The listing builds one solid part. Answer for the finished solid, in the listing's coordinates (mm). Coordinates: 2 decimals unless noted, no trailing zeros. Order: outer loops, then holes, each group sorted by start corner. A loop starts at its lowest first (then second) coordinate and runs counter-clockwise, first axis right, second up.
from build123d import *

# Parameters (mm, degrees)
F0_W     = 279.4
F0_H     = 101.6
F1_DEPTH = 12.7
F2_R     = 12.7
F4_D     = 7.9375
F6_D     = 7.9375
F8_D     = 12.7


with BuildPart() as f1:
    # F0 (on Front) → F1 (new body)
    with BuildSketch(Plane.XZ):
        with Locations((62.394057, 50.8)):
            Rectangle(F0_W, F0_H)
    extrude(amount=F1_DEPTH)

    # F2
    f2_edges = [f1.edges().sort_by_distance(p)[0] for p in [
        (-77.305943, -6.35, 101.6),
        (-77.305943, -6.35, 0),
        (202.094057, -6.35, 101.6),
        (202.094057, -6.35, 0),
    ]]
    fillet(f2_edges, radius=F2_R)

    # F4 (through all)
    with Locations(Plane.XZ.offset(12.7)):
        with Locations((62.394057, 50.8)):
            Hole(F4_D / 2)

    # F6 (through all)
    with Locations(Plane.XZ.offset(12.7)):
        with Locations((190.981557, 50.8), (-39.205943, 50.8)):
            Hole(F6_D / 2)

    # F8 (through all)
    with Locations(Plane.XZ.offset(12.7)):
        with Locations((-66.193443, 50.8)):
            Hole(F8_D / 2)


solid = f1.part
(1) Find section A-A on z = 50.8. Determine the outline of the cut face in (x, y), then the cut area to 3 significant figures.
(2) Given pin 1 Ø7 at (x, z) = (-39.21, 50.8) entering from +Y; pin 2 Ø10.5 at (x, z) = (62.39, 50.8) entering from +Y, each flat-ended and moving along its own axis, determine where each tip first touches the part or whether it passes through.
(3) Find the intervals of material crossed by probe 1 along X at (y, z) = (-8.25, 94); probe 2 along X at (y, z) = (-1.5, 6); probe 3 along Z at (x, y) = (-61, -8), in increasing order.
(4) The mould has two halves that part along Z. Classify faces 1 (the cylindrical face through (194.946, -6.261, 50.974)), 2 (the cylindrical face through (198.473, -6.439, 97.781)), 3 (the flat face through (-77.306, -6, 50)): pulls with the +Z half, pulls with the -Z half, needs draft (parallel to the pull), parting line crosses it, or undercut.
Resolved:
1. outline: (-77.31, -12.7) - (-72.54, -12.7) - (-72.54, 0) - (-77.31, 0) - close; (-59.84, -12.7) - (-43.17, -12.7) - (-43.17, 0) - (-59.84, 0) - close; (-35.24, -12.7) - (58.43, -12.7) - (58.43, 0) - (-35.24, 0) - close; (66.36, -12.7) - (187.01, -12.7) - (187.01, 0) - (66.36, 0) - close; (194.95, -12.7) - (202.09, -12.7) - (202.09, 0) - (194.95, 0) - close
1. area: 3,080 mm2
2. pin 1: passes through
2. pin 2: stops at y = 0
3. probe 1: x = -76.24 to 201.03
3. probe 2: x = -75.39 to 200.18
3. probe 3: z = 0 to 47.15, 54.45 to 101.6
4. face 1: undercut
4. face 2: pulls with the +Z half
4. face 3: needs draft
